Part model, mm, in its own coordinate system. Face numbers are marked on the shaded views. A direction names the side the tool comes from. Round coordinates to 2 decimals unless told otherwise and drop trailing zeros. Order: outer loops, then holes, each group sorted by start corner. A loop starts at its lowest first (then second) coordinate and runs counter-clockwise, first axis right, second up. Notation, with made-up numbers: (26.5, -1) - (76.5, -1) arc R31 cw to (76.5, 34) - close; hole circle Ø1 at (34.25, -15.5). An arc over 180 degrees is marked (long way). Answer as a JSON object with one key per item and string values.
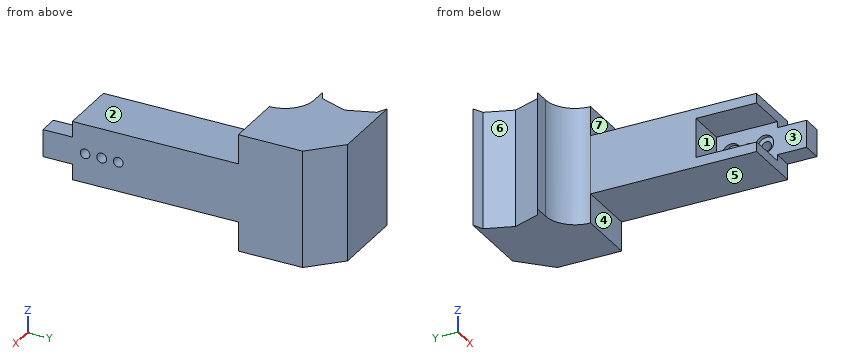
Autodesk Inventor part; units mm, degrees
ref_plane "Work Plane1" through (0, 0, -15) normal (0, 0, 1) x (1, 0, 0)
ref_plane "YZ Plane" through (0, 0, 0) normal (1, 0, 0) x (0, 1, 0)
ref_plane "XZ Plane" through (0, 0, 0) normal (0, 1, 0) x (-1, 0, 0)
sketch "Sketch1" plane through (0, 0, 0) normal (0, 0, 1) x (1, 0, 0)
  line L0 (0, 0) -> (25, 0)
  line L1 (25, 0) -> (25, 40)
  line L2 (25, 40) -> (0, 40)
  line L3 (0, 40) -> (0, 0)
  dimension "d1" = 25
  dimension "d2" = 40
  dimension "d3" = 25
extrude "Extrusion1" add sketch "Sketch1" against normal blind 30
sketch "Sketch2" plane through (25, 0, 0) normal (1, 0, 0) x (0, 0, -1)
  line L0 (0, 0) -> (30, 0)
  circle A0 centre (15, 6.56) radius 2.46
extrude "Extrusion2" cut sketch "Sketch2" against normal blind 30
sketch "Sketch3" plane through (0, 0, 0) normal (-1, 0, 0) x (0, 0, 1)
  line L0 (0, 0) -> (-30, 0)
  line L1 (-25.05, 0) -> (-4.95, 0)
  line L2 (-4.95, 0) -> (-4.95, 33.12)
  line L3 (-4.95, 33.12) -> (-25.05, 33.12)
  line L4 (-25.05, 33.12) -> (-25.05, 0)
  dimension "d11" = 20.1
extrude "Extrusion3" cut sketch "Sketch3" against normal blind 20
sketch "Sketch4" plane through (0, 0, 0) normal (0, -1, 0) x (1, 0, 0)
  line L0 (20, -4.95) -> (20, -25.05)
  line L1 (20, -15) -> (25, -15)
  line L2 (25, 0) -> (25, -30)
  line L3 (20, -8.025) -> (25, -8.025)
  line L4 (25, -8.025) -> (25, -21.975)
  line L5 (25, -21.975) -> (20, -21.975)
  line L6 (20, -21.975) -> (20, -8.025)
  line L7 (20, -8.025) -> (25, -21.975) construction
  line L8 (25, -8.025) -> (20, -21.975) construction
  line L9 (25, -12.54) -> (25, -17.46)
  point P0 (0, 0)
  point P1 (22.5, -15)
  dimension "d14" = 13.95
extrude "Extrusion4" add sketch "Sketch4" along normal blind 15
sketch "Sketch5" plane through (20, 0, 0) normal (-1, 0, 0) x (0, 0, 1)
  circle A0 centre (-15, 6.56) radius 2.46
  circle A1 centre (-15, 6.56) radius 4.7025
  circle A2 centre (-15, 6.56) radius 2.46
  circle A3 centre (-15, 6.56) radius 2.46
  point P0 (0, 0)
  dimension "d17" = 9.405
extrude "Extrusion5" cut sketch "Sketch5" against normal blind 2.1
sketch "Sketch6" plane through (25, 0, 0) normal (1, 0, 0) x (0, 0, -1)
  circle A0 centre (15, 6.56) radius 4.7025
  line L0 (15, 6.56) -> (15, 23.56)
  circle A1 centre (15, 23.56) radius 2.46
  point P0 (0, 0)
  dimension "d20" = 17
  dimension "d21" = 4.92
extrude "Extrusion6" cut sketch "Sketch6" against normal blind 10 contours A1
sketch "Sketch7" plane through (20, 0, 0) normal (-1, 0, 0) x (0, 0, 1)
  circle A0 centre (-15, 23.56) radius 2.46
  circle A1 centre (-15, 23.56) radius 4.7025
  point P0 (0, 0)
  dimension "d24" = 9.405
extrude "Extrusion7" cut sketch "Sketch7" against normal blind 2.1
sketch "Sketch9" plane through (25, 0, 0) normal (1, 0, 0) x (0, 0, -1)
  circle A0 centre (15, 6.56) radius 2.46
  circle A1 centre (15, 6.56) radius 2.46
  circle A2 centre (15, 23.56) radius 2.46
  circle A3 centre (15, 23.56) radius 2.46
  line L0 (30, 40) -> (30, 0)
  line L1 (30, 0) -> (30, 40)
  line L2 (30, 40) -> (0, 40)
  line L3 (0, 40) -> (0, 0)
  line L4 (0, 0) -> (8.025, 0)
  line L5 (21.975, 0) -> (21.975, -15)
  line L6 (21.975, -15) -> (8.025, -15)
  line L7 (8.025, -15) -> (8.025, 0)
  line L8 (0, 0) -> (8.025, 0)
  line L9 (21.975, 0) -> (30, 0)
extrude "Extrusion8" add sketch "Sketch9" along normal blind 5
sketch "Sketch10" plane through (0, 40, 0) normal (0, 1, 0) x (1, 0, 0)
  line L0 (0, 30) -> (30, 30)
  line L1 (30, 0) -> (0, 0)
  line L2 (0, 30) -> (30, 30)
  line L3 (30, 30) -> (30, 0)
  line L4 (30, 0) -> (0, 0)
  line L5 (0, 0) -> (0, 30)
extrude "Extrusion9" add sketch "Sketch10" along normal blind 30
sketch "Sketch12" plane through (30, 0, 0) normal (1, 0, 0) x (0, 0, -1)
  circle A0 centre (15, 6.56) radius 2.46
  line L0 (15, 6.56) -> (15, 15.06)
  circle A1 centre (15, 15.06) radius 2.525
  point P0 (0, 0)
  dimension "d31" = 8.5
  dimension "d33" = 5.05
extrude "Extrusion10" cut sketch "Sketch12" against normal blind 30 contours A1
sketch "Sketch14" plane through (0, 0, 0) normal (0, 0, 1) x (1, 0, 0)
  line L0 (30, 70) -> (0, 70)
  line L1 (0, 70) -> (0, 85)
  line L2 (-15, 100) -> (-23, 100)
  line L3 (30, 0) -> (30, 70)
  line L4 (30, 118) -> (30, 70)
  arc A0 (0, 85) -> (-15, 100) centre (-15, 85) ccw
  line L5 (30, 105) -> (30, 100)
  line L6 (-23, 133) -> (15, 133)
  line L7 (-18, 130.5) -> (-23, 133)
  line L8 (-18, 130.5) -> (-13, 116.5)
  line L9 (-18, 102.5) -> (-23, 100)
  line L10 (-18, 102.5) -> (-13, 116.5)
  line L11 (30, 118) -> (15, 133)
  point P0 (0, 0)
  point P1 (0, 100)
  dimension "d47" = 30
  dimension "d54" = 15
extrude "Extrusion12" add sketch "Sketch14" against normal blind 30
sketch "Sketch15" plane through (0, 0, -25.05) normal (-1, 0, 0) x (0, 0, 1)
  line L0 (0, 33.12) -> (20.1, 33.12)
  line L1 (20.1, 33.12) -> (20.1, 0)
  line L2 (0, 33.12) -> (20.1, 33.12)
  line L3 (20.1, 33.12) -> (20.1, 31.1)
  line L4 (20.1, 31.1) -> (0, 31.1)
  line L5 (0, 31.1) -> (0, 33.12)
  point P0 (25.05, 0)
  dimension "d57" = 2.02
extrude "Extrusion13" add sketch "Sketch15" against normal blind 20
sketch "Sketch21" plane through (0, 0, 0) normal (0, 0, 1) x (1, 0, 0)
  arc A0 (0, 85) -> (-15, 100) centre (-15, 85) ccw
  arc A1 (0, 85) -> (-15, 100) centre (-15, 85) ccw
  line L0 (-15, 100) -> (-23, 100)
  line L1 (-15, 100) -> (-23, 100)
  line L2 (-23, 100) -> (-18, 102.5)
  line L3 (-23, 100) -> (-18, 102.5)
  line L4 (-18, 102.5) -> (-13, 116.5)
  line L5 (-18, 102.5) -> (-13, 116.5)
  line L6 (-13, 116.5) -> (-18, 130.5)
  line L7 (-13, 116.5) -> (-18, 130.5)
  line L8 (-18, 130.5) -> (-23, 133)
  line L9 (-18, 130.5) -> (-23, 133)
  line L10 (-23, 133) -> (15, 133)
  line L11 (-23, 133) -> (15, 133)
  line L12 (15, 133) -> (30, 118)
  line L13 (15, 133) -> (30, 118)
  line L14 (0, 85) -> (30, 85)
  line L15 (30, 85) -> (30, 118)
  point P0 (0, 0)
extrude "Extrusion14" add sketch "Sketch21" along normal blind 15
ref_plane "Work Plane1" through (0, 0, -15) normal (0, 0, 1) x (1, 0, 0)
mirror "Mirror1" about plane through (0, 0, -15) normal (0, 0, 1) of "Extrusion14"
properties part number "28mm_x_60mm"
Item 1: Two-plate mould, pull along Z, no slides. Class the marked faces 1, 2, 3 and 4: pulls with the +Z half, pulls with the -Z half, needs draft (parallel to the pull), parting line crosses it, or undercut.
Taken from the geometry:
{"face 1": "undercut", "face 2": "pulls with the +Z half", "face 3": "undercut", "face 4": "needs draft"}
Item 2: Cut at A-A (z = -15). State how many separate pieces and enclosed holes the cut face has, plus the area to 3 significant figures.
Taken from the geometry:
{"separate pieces": "4", "enclosed holes": "0", "area": "3,820 mm2"}
Item 3: Cut at B-B (x = 25.5). Write the cut outline in (y, z) (3 decimals).
Taken from the geometry:
{"outline": "(-15, -21.975) - (0, -21.975) - (0, -30) - (85, -30) - (85, -45) - (122.5, -45) - (122.5, 15) - (85, 15) - (85, 0) - (0, 0) - (0, -8.025) - (-15, -8.025) - close; hole circle Ø4.92 at (6.56, -15); hole circle Ø5.05 at (15.06, -15); hole circle Ø4.92 at (23.56, -15)"}
Item 4: Cut at D-D (x = 6). Write the cut outline in (y, z).
Taken from the geometry:
{"outline": "(0, -30) - (85, -30) - (85, -45) - (133, -45) - (133, 15) - (85, 15) - (85, 0) - (0, 0) - (0, -4.95) - (31.1, -4.95) - (31.1, -25.05) - (0, -25.05) - close"}
Item 5: Tool access for the marked faces 5, 6 and 7: list every direction of +Z, -Z, +X, -X, +Y, -Y with a clear straight run to the whole face (end or side of a thin tool).
Taken from the geometry:
{"face 5": "-Z, +X, -X, -Y", "face 6": "+Z, -Z, -X", "face 7": "+Z, +X, -X, -Y"}
Item 6: Drop flat-ended pins along their axis: P1, Ø6.5, axis at x = 18.5, z = -25.5, coming from the -Y side; P2, Ø4, axis at y = 8.5, z = 0.5, coming from the -X side; P3, Ø3, axis at y = 9, z = -13, coming from the -X side. Give the stop position or say it passes through.
Taken from the geometry:
{"P1": "y = 0", "P2": "x = 0", "P3": "x = 22.1"}
Item 7: Probe L1, parallel to Y at x = 27, z = -15 (3 decimals); L2, parallel to Y at x = 25.25, z = -15 (3 decimals); L3, parallel to Z at x = 5.5, y = 19.5. List the from-to ranges inside material, lowest first. Write a range as from..to.
Taken from the geometry:
{"L1": "-15..4.1, 9.02..12.535, 17.585..21.1, 26.02..121", "L2": "-15..4.1, 9.02..12.535, 17.585..21.1, 26.02..122.75", "L3": "-30..-25.05, -4.95..0"}
Item 8: Cut at C-C (y = 23.56). Write the cut outline in (x, z).
Taken from the geometry:
{"outline": "(0, -30) - (30, -30) - (30, -17.46) - (22.1, -17.46) - (22.1, -19.7) - (20, -19.7) - (20, -25.05) - (0, -25.05) - close; (0, -4.95) - (20, -4.95) - (20, -10.3) - (22.1, -10.3) - (22.1, -12.54) - (30, -12.54) - (30, 0) - (0, 0) - close"}
